Build history of the part. All positions in model axes, mm. Face numbers are marked on the shaded views. A direction names the side the tool comes from. Round coordinates to 2 decimals unless told otherwise and drop trailing zeros. Order: outer loops, then holes, each group sorted by start corner. A loop starts at its lowest first (then second) coordinate and runs counter-clockwise, first axis right, second up. Notation, with made-up numbers: M -12.75,-0.5 L 27.25,-0.5 A7 ccw 27.25,8.5 Z; hole C 32,-25 d3. An arc over 180 degrees is marked long. One line per item, written item: value. Start each with the question number.
Item 1: Band-saw the part on D-D, the plane y = -22. Give the number of separate pieces and of enclosed holes in the cut face, then the cut area to 3 significant figures.
Item 2: Band-saw the part on B-B, the plane x = -1.5. Write the cut outline in (y, z), then the cut area to 3 significant figures.
Item 3: Pin check, flat tips, straight feed: pin 1 (2 mm diameter, centred on x = 12.5, y = 24.5, fed in from +Z); pin 2 (2 mm diameter, centred on y = 21, z = 12, fed in from -X); pin 3 (2.5 mm diameter, centred on y = -17, z = 67.5, fed in from +X). Stop position of each tip, or through.
Item 4: Probe L1, parallel to X at y = 0, z = 55.25; L2, parallel to Z at x = 2.5, y = 16; L3, parallel to X at y = 0, z = 19.5. List the from-to ranges inside material, lowest first.
Item 5: Tool access for the marked faces 4, 5, 6, 7 and 8: list every direction of +Z, -Z, +X, -X, +Y, -Y with a clear straight run to the whole face (end or side of a thin tool).
Item 6: Band-saw the part on A-A, the plane x = 24.5. Write the cut outline in (y, z), then the cut area to 3 significant figures.
Item 7: Band-saw the part on C-C, the plane y = 5. Write the cut outline in (x, z), then the cut area to 3 significant figures.
Item 8: Two-plate mould, pull along Z, no slides. Class the marked faces 1, 2 and 3: +Z half, -Z half, draft (parallel to the pull), parting line (faces both ways), or undercut.
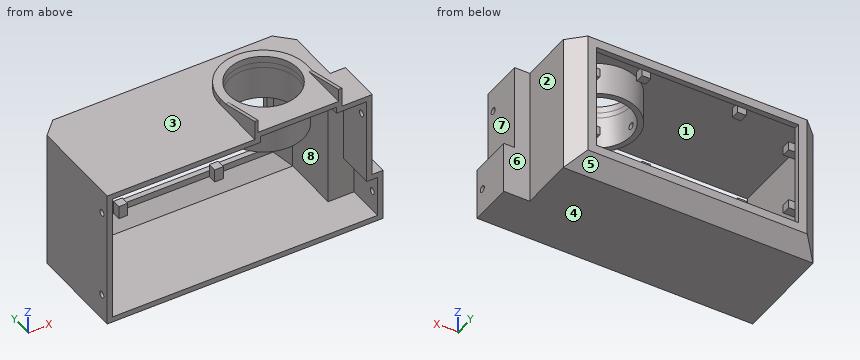
```python
from build123d import *

# Parameters (mm, degrees)
BOSS_EXTRUDE1_DEPTH = 64
SKETCH2_R           = 20
SKETCH2_R_2         = 16
BOSS_EXTRUDE2_DEPTH = 3
CHAMFER1_SIZE       = 7
BOSS_EXTRUDE3_REACH = 97.902
SKETCH4_W           = 1.5
SKETCH4_H           = 22
BOSS_EXTRUDE4_DEPTH = 6
CUT_EXTRUDE1_DEPTH  = 104.097041665
SKETCH6_W           = 5
SKETCH6_H           = 40
CUT_EXTRUDE2_DEPTH  = 102.908046787
SHELL1_START        = 2.5
SHELL1_DEPTH        = 59
SHELL1_2_OUTLINE_W  = 5
SHELL1_2_OUTLINE_H  = 17.5
SHELL1_2_DEPTH      = 19
SHELL1_START_2      = 61.5
SHELL1_3_DEPTH      = 3
SHELL1_START_3      = 10.935028843
SHELL1_4_DEPTH      = 2.5
CUT_EXTRUDE3_REACH  = 95.831
SKETCH7_R           = 16
BOSS_EXTRUDE5_START = 15
SKETCH8_R           = 16
BOSS_EXTRUDE5_DEPTH = 15
CUT_EXTRUDE4_REACH  = 111.842
SKETCH9_W           = 93
SKETCH9_H           = 49
SKETCH10_W          = 6
SKETCH10_H          = 4
SKETCH10_W_2        = 4
SKETCH10_H_2        = 6
BOSS_EXTRUDE6_DEPTH = 4
SKETCH11_R          = 1.5
CUT_EXTRUDE5_DEPTH  = 149.7749979
SKETCH12_R          = 1.55
CUT_EXTRUDE6_DEPTH  = 44


with BuildPart() as part:
    # Sketch1 → Boss-Extrude1 (new body)
    with BuildSketch(Plane.XY):
        Polygon((63.5, -26), (63.5, -6), (51.5, -6), (51.5, 26), (-63.5, 26), (-63.5, -26), align=None)
    extrude(amount=BOSS_EXTRUDE1_DEPTH)

    # Sketch2 → Boss-Extrude2 (add)
    with BuildSketch(Plane.XY.offset(64)):
        with Locations((24.5, 0)):
            Circle(SKETCH2_R)
        with Locations((24.5, 0)):
            Circle(SKETCH2_R_2, mode=Mode.SUBTRACT)
    extrude(amount=BOSS_EXTRUDE2_DEPTH)

    # Chamfer1
    chamfer1_edges = [part.edges().sort_by_distance(p)[0] for p in [
        (-63.5, 26, 32),
        (51.5, 26, 32),
        (-6, 26, 0),
    ]]
    chamfer(chamfer1_edges, length=CHAMFER1_SIZE)

    # Sketch3 → Boss-Extrude3 (add, up to next)
    with BuildSketch(Plane.XY.offset(67), mode=Mode.PRIVATE) as boss_extrude3_sk1:
        with BuildLine():
            ThreePointArc((6.5, -8.717797887), (5.00641131, -4.472135955), (4.5, 0))
            Line((4.5, 0), (4.5, -26))
            Line((4.5, -26), (6.5, -26))
            Line((6.5, -26), (6.5, -8.717797887))
        make_face()
    boss_extrude3_tool1 = extrude(boss_extrude3_sk1.sketch, amount=-BOSS_EXTRUDE3_REACH, mode=Mode.PRIVATE) - part.part
    # Sketch3 → Boss-Extrude3 (add, up to next)
    with BuildSketch(Plane.XY.offset(67), mode=Mode.PRIVATE) as boss_extrude3_sk2:
        with BuildLine():
            Line((44.5, -26), (44.5, 0))
            ThreePointArc((44.5, 0), (43.99358869, -4.472135955), (42.5, -8.717797887))
            Line((42.5, -8.717797887), (42.5, -26))
            Line((42.5, -26), (44.5, -26))
        make_face()
    boss_extrude3_tool2 = extrude(boss_extrude3_sk2.sketch, amount=-BOSS_EXTRUDE3_REACH, mode=Mode.PRIVATE) - part.part
    # Sketch3 → Boss-Extrude3 (add, up to next)
    with BuildSketch(Plane.XY.offset(67), mode=Mode.PRIVATE) as boss_extrude3_sk3:
        with BuildLine():
            ThreePointArc((42.5, -8.717797887), (24.5, -20), (6.5, -8.717797887))
            Line((6.5, -8.717797887), (6.5, -26))
            Line((6.5, -26), (42.5, -26))
            Line((42.5, -26), (42.5, -8.717797887))
        make_face()
    boss_extrude3_tool3 = extrude(boss_extrude3_sk3.sketch, amount=-BOSS_EXTRUDE3_REACH, mode=Mode.PRIVATE) - part.part
    add(boss_extrude3_tool1.solids().sort_by_distance((5.442676, -15.832473, 67))[0])
    add(boss_extrude3_tool2.solids().sort_by_distance((43.557324, -15.832473, 67))[0])
    add(boss_extrude3_tool3.solids().sort_by_distance((24.5, -20.87134, 67))[0])

    # Sketch4 → Boss-Extrude4 (add)
    with BuildSketch(Plane.XY.offset(67)):
        with Locations((43.75, -15)):
            Rectangle(SKETCH4_W, SKETCH4_H)
        with Locations((5.25, -15)):
            Rectangle(SKETCH4_W, SKETCH4_H)
    extrude(amount=BOSS_EXTRUDE4_DEPTH)

    # Sketch5 → Cut-Extrude1 (cut, through all)
    with BuildSketch(Plane.ZY.offset(-4.5)):
        Polygon((67, -4), (73, -26), (73, -4), align=None)
    extrude(amount=-CUT_EXTRUDE1_DEPTH, mode=Mode.SUBTRACT)

    # Sketch6 → Cut-Extrude2 (cut, through all)
    with BuildSketch(Plane(origin=(0, -6, 0), x_dir=(1, 0, 0), z_dir=(0, 1, 0))):
        with Locations((61, -44)):
            Rectangle(SKETCH6_W, SKETCH6_H)
    extrude(amount=-CUT_EXTRUDE2_DEPTH, mode=Mode.SUBTRACT)

    # Shell1: read off the stored shape, not the designer's step
    # Shell1 outline → Shell1 (cut)
    with BuildSketch(Plane.XY.offset(SHELL1_START)):
        Polygon((56, -8.5), (49, -8.5), (49, 17.964466094), (43.464466094, 23.5), (-55.464466094, 23.5), (-61, 17.964466094), (-61, -26), (56, -26), align=None)
    extrude(amount=SHELL1_DEPTH, mode=Mode.SUBTRACT)

    # Shell1 2 outline → Shell1 2 (cut)
    with BuildSketch(Plane.XY.offset(SHELL1_START)):
        with Locations((58.5, -17.25)):
            Rectangle(SHELL1_2_OUTLINE_W, SHELL1_2_OUTLINE_H)
    extrude(amount=SHELL1_2_DEPTH, mode=Mode.SUBTRACT)

    # Shell1 3 outline → Shell1 3 (cut)
    with BuildSketch(Plane.XY.offset(SHELL1_START_2)):
        with BuildLine():
            Line((7, -26), (42, -26))
            Line((42, -26), (42, -6))
            ThreePointArc((42, -6), (24.5, -18.5), (7, -6))
            Line((7, -6), (7, -26))
        make_face()
    extrude(amount=SHELL1_3_DEPTH, mode=Mode.SUBTRACT)

    # Shell1 4 outline → Shell1 4 (add)
    with BuildSketch(Plane(origin=(0, 0, 0), x_dir=(1, 0, 0), z_dir=(0, 0.707106781186545, -0.70710678118655)).offset(SHELL1_START_3)):
        Polygon((43.464466094, -22.298989873), (49, -14.470562748), (-61, -14.470562748), (-55.464466094, -22.298989873), align=None)
    extrude(amount=SHELL1_4_DEPTH)

    # Sketch7 → Cut-Extrude3 (cut, up to next)
    with BuildSketch(Plane.XY.offset(64), mode=Mode.PRIVATE) as cut_extrude3_sk1:
        with Locations((24.5, 0)):
            Circle(SKETCH7_R)
    cut_extrude3_tool1 = extrude(cut_extrude3_sk1.sketch, amount=-CUT_EXTRUDE3_REACH, mode=Mode.PRIVATE) & part.part
    add(cut_extrude3_tool1.solids().sort_by_distance((24.5, 0, 64))[0], mode=Mode.SUBTRACT)

    # Sketch8 → Boss-Extrude5 (add)
    with BuildSketch(Plane(origin=(0, 0, 61.5), x_dir=(-1, 0, 0), z_dir=(0, 0, -1)).offset(BOSS_EXTRUDE5_START)):
        with BuildLine():
            ThreePointArc((-6, 0), (-27.541381265, 18.248287591), (-42, -6))
            ThreePointArc((-42, -6), (-24.5, -18.5), (-7, -6))
            ThreePointArc((-7, -6), (-6.251712409, -3.041381265), (-6, 0))
        make_face()
        with Locations((-24.5, 0)):
            Circle(SKETCH8_R, mode=Mode.SUBTRACT)
    extrude(amount=-BOSS_EXTRUDE5_DEPTH)

    # Sketch9 → Cut-Extrude4 (cut, up to next)
    with BuildSketch(Plane(origin=(0, 26, 0), x_dir=(1, 0, 0), z_dir=(0, 1, 0)), mode=Mode.PRIVATE) as cut_extrude4_sk1:
        with Locations((-6, -35.5)):
            Rectangle(SKETCH9_W, SKETCH9_H)
    cut_extrude4_tool1 = extrude(cut_extrude4_sk1.sketch, amount=-CUT_EXTRUDE4_REACH, mode=Mode.PRIVATE) & part.part
    add(cut_extrude4_tool1.solids().sort_by_distance((-6, 26, 35.5))[0], mode=Mode.SUBTRACT)

    # Sketch10 → Boss-Extrude6 (add)
    with BuildSketch(Plane.XZ.offset(-23.5)):
        with Locations((-52.464466094, 50)):
            Rectangle(SKETCH10_W, SKETCH10_H)
        with Locations((-52.464466094, 21)):
            Rectangle(SKETCH10_W, SKETCH10_H)
        with Locations((40.464466094, 21)):
            Rectangle(SKETCH10_W, SKETCH10_H)
        with Locations((40.464466094, 50)):
            Rectangle(SKETCH10_W, SKETCH10_H)
        with Locations((-28, 11.035533906)):
            Rectangle(SKETCH10_W_2, SKETCH10_H_2)
        with Locations((16, 11.035533906)):
            Rectangle(SKETCH10_W_2, SKETCH10_H_2)
        with Locations((16, 59.964466094)):
            Rectangle(SKETCH10_W_2, SKETCH10_H_2)
        with Locations((-28, 59.964466094)):
            Rectangle(SKETCH10_W_2, SKETCH10_H_2)
    extrude(amount=BOSS_EXTRUDE6_DEPTH)

    # Sketch11 → Cut-Extrude5 (cut, through all)
    with BuildSketch(Plane.ZY.offset(63.5)):
        with Locations(Location((53, -22, 0), (0, 0, 270))):
            Circle(SKETCH11_R)
        with Locations((12, -22)):
            Circle(SKETCH11_R)
    extrude(amount=-CUT_EXTRUDE5_DEPTH, mode=Mode.SUBTRACT)

    # Sketch12 → Cut-Extrude6 (cut)
    with BuildSketch(Plane(origin=(0, 0, 0), x_dir=(0, 0, -1), z_dir=(1, 0, 0))):
        with Locations(Location((-51.5, 0, 0), (0, 0, 180))):
            Circle(SKETCH12_R)
    extrude(amount=CUT_EXTRUDE6_DEPTH, mode=Mode.SUBTRACT)


solid = part.part
```
Output:
1. separate pieces: 4
1. enclosed holes: 0
1. area: 930 mm²
2. outline: M -26,0 L 19,0 L 26,7 L 26,11 L 23.5,11 L 23.5,8.04 L 17.96,2.5 L -26,2.5 Z; M -26,61.5 L 23.5,61.5 L 23.5,60 L 26,60 L 26,64 L -26,64 Z
2. area: 276 mm²
3. pin 1: stops at z = 64
3. pin 2: stops at x = -62.5
3. pin 3: stops at x = 44.5
4. L1: x = -63.5 to -61, 6 to 8.5, 40.5 to 43, 49 to 51.5
4. L2: z = 0 to 2.5, 61.5 to 64
4. L3: x = -63.5 to -61, 49 to 51.5
5. face 4: -Z, +X, -X, +Y, -Y
5. face 5: -Z, +X, -X, +Y
5. face 6: +Z, -Z, +X, +Y
5. face 7: +Z, +X, +Y, -Y
5. face 8: -Y
6. outline: M -26,0 L 19,0 L 26,7 L 26,11 L 23.5,11 L 23.5,8.04 L 17.96,2.5 L -26,2.5 Z; M -26,64.5 L -18.5,64.5 L -18.5,46.5 L -16,46.5 L -16,67 L -26,67 Z; M 16,46.5 L 18.5,46.5 L 18.5,61.5 L 23.5,61.5 L 23.5,60 L 26,60 L 26,64 L 20,64 L 20,67 L 16,67 Z
6. area: 290 mm²
7. outline: M -63.5,0 L 51.5,0 L 51.5,64 L 43.86,64 L 43.86,67 L 39.7,67 L 39.7,46.5 L 42.31,46.5 L 42.31,61.5 L 49,61.5 L 49,2.5 L -61,2.5 L -61,61.5 L 6.69,61.5 L 6.69,46.5 L 9.3,46.5 L 9.3,67 L 5.14,67 L 5.14,64 L -63.5,64 Z
7. area: 897 mm²
8. face 1: undercut
8. face 2: draft
8. face 3: +Z half
